Model file for the job. Use its own axes, mm. A direction names the side the tool comes from. Round coordinates to 2 decimals unless told otherwise and drop trailing zeros. Loops run counter-clockwise (first coordinate to the right, second up) from the corner with the lowest first, then second, coordinate; pieces in that order, holes last. Notation, with made-up numbers: M -35.5,-31 L 0.5,-31 A27 cw 0.5,4 Z; hole C 84,27.5 d11. An arc over 180 degrees is marked long. Use a Markdown table: item, result. Add a question column.
Q1. Probe line 1 (Y direction, x = 0, z = -74.25); line 2 (Y direction, x = 0.5, z = -64.75); line 3 (Z direction, x = -8, y = -16.25). List the from-to ranges inside material, lowest first. Write a range as from..to.
Q2. Pin check, flat tips, straight feed: pin 1 (4 mm diameter, centred on y = -23, z = -63, fed in from -X); pin 2 (1.5 mm diameter, centred on x = 5.5, z = -75, fed in from -Y); pin 3 (3 mm diameter, centred on y = -17, z = -65.5, fed in from +X). Stop position of each tip, or through.
Q3. Cut at D-D (z = -66.25). Give the cut face in (x, y) (1 decimal).
Q4. Cut at B-B (y = -22.75). Give the cut face in (x, z), plus the area to 3 significant figures.
Q5. Tool access for faces 1 (the face through (3.5, -27.53, -80.03)), 2 (the face through (1, -27, -81.458)), 3 (the face through (6, -15, -66.738)): list every direction of +Z, -Z, +X, -X, +Y, -Y with a clear straight run to the whole face (end or side of a thin tool).
Q6. Cut at C-C (x = -8). Give the cut face in (y, z).
Q7. Cut at A-A (x = 0). Give the cut face in (y, z), plus the area to 3 significant figures.
from build123d import *


with BuildPart() as part:
    # Sketch1 → Revolve1 (revolve)
    with BuildSketch(Plane(origin=(0, 0, 0), x_dir=(0, 0, -1), z_dir=(1, 0, 0)), mode=Mode.PRIVATE) as revolve1_sk:
        with BuildLine():
            Line((60.7822, -26.811732), (81.4578, -26.811732))
            Line((81.4578, -26.811732), (81.4578, -28.551632))
            Line((81.4578, -28.551632), (78.639993039, -28.551632))
            ThreePointArc((78.639993039, -28.551632), (77.1926569, -29.920339878), (75.5015, -30.973018125))
            Line((75.5015, -30.973018125), (75.5015, -33.555432))
            Line((75.5015, -33.555432), (66.7385, -33.555432))
            Line((66.7385, -33.555432), (66.7385, -30.973018125))
            ThreePointArc((66.7385, -30.973018125), (65.0473431, -29.920339878), (63.600006961, -28.551632))
            Line((63.600006961, -28.551632), (60.7822, -28.551632))
            Line((60.7822, -28.551632), (60.7822, -26.811732))
        make_face()
    revolve(revolve1_sk.sketch.rotate(Axis((0, -22.049232, -82.136173087), (0, 0, -1)), 270), axis=Axis((0, -22.049232, -82.136173087), (0, 0, -1)))


solid = part.part
Checked values:
| question | item | result |
|---|---|---|
| 1 | line 1 | y = -33.56..-26.81, -17.29..-10.54 |
| 1 | line 2 | y = -29.67..-26.79, -17.31..-14.43 |
| 1 | line 3 | z = -75.5..-66.74 |
| 2 | pin 1 | stops at x = -7.79 |
| 2 | pin 2 | stops at y = -32.53 |
| 2 | pin 3 | stops at x = 10.71 |
| 3 | outline | C 0,-22 d17.3; hole C 0,-22 d9.5 |
| 4 | outline | M -11.48,-75.5 L -8.9,-75.5 A9.92 ccw -6.46,-78.64 L -6.46,-81.46 L -4.71,-81.46 L -4.71,-60.78 L -6.46,-60.78 L -6.46,-63.6 A9.92 ccw -8.9,-66.74 L -11.48,-66.74 Z; M 4.71,-81.46 L 6.46,-81.46 L 6.46,-78.64 A9.92 ccw 8.9,-75.5 L 11.48,-75.5 L 11.48,-66.74 L 8.9,-66.74 A9.92 ccw 6.46,-63.6 L 6.46,-60.78 L 4.71,-60.78 Z |
| 4 | area | 178 mm^2 |
| 5 | face 1 | -Z |
| 5 | face 2 | -Z, +X, -X, +Y, -Y |
| 5 | face 3 | +Z |
| 6 | outline | M -30.32,-75.5 L -26,-75.5 A5.9 ccw -18.1,-75.5 L -13.78,-75.5 L -13.78,-66.74 L -18.1,-66.74 A5.9 ccw -26,-66.74 L -30.32,-66.74 Z |
| 7 | outline | M -33.56,-75.5 L -30.97,-75.5 A9.94 ccw -28.55,-78.64 L -28.55,-81.46 L -26.81,-81.46 L -26.81,-60.78 L -28.55,-60.78 L -28.55,-63.6 A9.94 ccw -30.97,-66.74 L -33.56,-66.74 Z; M -17.29,-81.46 L -15.55,-81.46 L -15.55,-78.64 A9.94 ccw -13.13,-75.5 L -10.54,-75.5 L -10.54,-66.74 L -13.13,-66.74 A9.94 ccw -15.55,-63.6 L -15.55,-60.78 L -17.29,-60.78 Z |
| 7 | area | 177 mm^2 |
